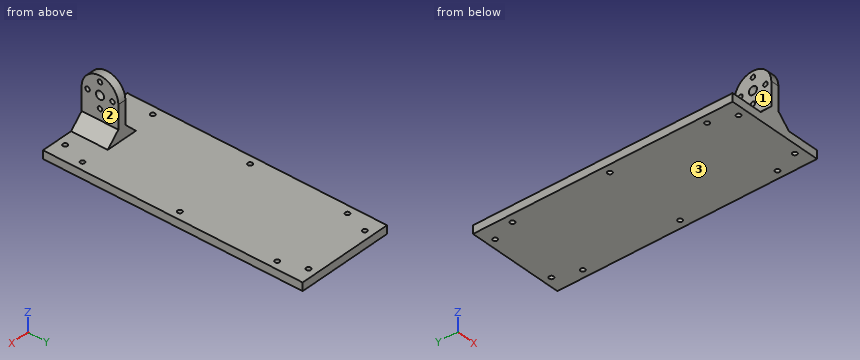
from build123d import *

# Parameters (mm, degrees)
SKETCH1_W           = 76.2
SKETCH1_H           = 203.2
BOSS_EXTRUDE1_DEPTH = 6.35
SKETCH2_W           = 6.35
SKETCH2_H           = 28.702
BOSS_EXTRUDE2_DEPTH = 44.45
SKETCH3_R           = 3.175
CUT_EXTRUDE1_DEPTH  = 6.35
SKETCH4_R           = 1.778
CUT_EXTRUDE2_DEPTH  = 6.35
CIRPATTERN1_COUNT   = 4
CUT_EXTRUDE3_DEPTH  = 6.35
SKETCH6_R           = 1.778
CUT_EXTRUDE4_DEPTH  = 6.35
BOSS_EXTRUDE3_DEPTH = 28.702


with BuildPart() as part:
    # Sketch1 → Boss-Extrude1 (new body)
    with BuildSketch(Plane.XY):
        with Locations((38.1, 101.6)):
            Rectangle(SKETCH1_W, SKETCH1_H)
    extrude(amount=BOSS_EXTRUDE1_DEPTH)

    # Sketch2 → Boss-Extrude2 (add)
    with BuildSketch(Plane.XY.offset(6.35)):
        with Locations((38.1, 14.351)):
            Rectangle(SKETCH2_W, SKETCH2_H)
    extrude(amount=BOSS_EXTRUDE2_DEPTH)

    # Sketch3 → Cut-Extrude1 (cut)
    with BuildSketch(Plane(origin=(41.275, 0, 0), x_dir=(0, 0, -1), z_dir=(1, 0, 0))):
        with Locations((-34.154615714, 14.351)):
            Circle(SKETCH3_R)
    extrude(amount=-CUT_EXTRUDE1_DEPTH, mode=Mode.SUBTRACT)

    # Sketch4 → Cut-Extrude2 (cut)
    with BuildSketch(Plane(origin=(41.275, 0, 0), x_dir=(0, 0, -1), z_dir=(1, 0, 0))):
        with Locations((-43.933615714, 14.351)):
            Circle(SKETCH4_R)
    cut_extrude2 = extrude(amount=-CUT_EXTRUDE2_DEPTH, mode=Mode.SUBTRACT)

    # CirPattern1: Cut-Extrude2 ×4 about axis
    cirpattern1_axis = Axis((0, 14.351, 34.154615714), (1, 0, 0))
    for i in range(1, CIRPATTERN1_COUNT):
        add(cut_extrude2.rotate(cirpattern1_axis, i * 360 / CIRPATTERN1_COUNT), mode=Mode.SUBTRACT)

    # Sketch5 → Cut-Extrude3 (cut)
    with BuildSketch(Plane(origin=(41.275, 0, 0), x_dir=(0, 0, -1), z_dir=(1, 0, 0))):
        with BuildLine():
            ThreePointArc((-34.154615714, 0), (-48.505615714, 14.351), (-34.154615714, 28.702))
            Line((-34.154615714, 28.702), (-50.8, 28.702))
            Line((-50.8, 28.702), (-50.8, 0))
            Line((-50.8, 0), (-34.154615714, 0))
        make_face()
    extrude(amount=-CUT_EXTRUDE3_DEPTH, mode=Mode.SUBTRACT)

    # Sketch6 → Cut-Extrude4 (cut)
    with BuildSketch(Plane(origin=(0, 0, 0), x_dir=(-1, 0, 0), z_dir=(0, 0, -1))):
        with Locations((-63.5, 6.35)):
            Circle(SKETCH6_R)
        with Locations((-12.7, 6.35)):
            Circle(SKETCH6_R)
        with Locations((-6.35, 177.8)):
            Circle(SKETCH6_R)
        with Locations((-6.35, 25.4)):
            Circle(SKETCH6_R)
        with Locations((-69.85, 25.4)):
            Circle(SKETCH6_R)
        with Locations((-69.85, 177.8)):
            Circle(SKETCH6_R)
        with Locations((-63.5, 196.85)):
            Circle(SKETCH6_R)
        with Locations((-12.7, 196.85)):
            Circle(SKETCH6_R)
        with Locations((-6.35, 101.6)):
            Circle(SKETCH6_R)
        with Locations((-69.85, 101.6)):
            Circle(SKETCH6_R)
    extrude(amount=-CUT_EXTRUDE4_DEPTH, mode=Mode.SUBTRACT)

    # Sketch8 → Boss-Extrude3 (add)
    with BuildSketch(Plane.XZ):
        Polygon((41.275, 6.35), (41.275, 15.875), (50.8, 6.35), align=None)
        Polygon((34.925, 6.35), (34.925, 15.875), (25.4, 6.35), align=None)
    extrude(amount=-BOSS_EXTRUDE3_DEPTH)


solid = part.part
Work out the finished part from the listing and answer in its coordinate system (mm). Face numbers are marked on the shaded views. A direction names the side the tool comes from. Coordinates: 2 decimals unless noted, no trailing zeros. Write each loop counter-clockwise with the first axis right and the second up, starting at its lowest first coordinate (ties: lowest second). Pieces come first, ordered by that corner, then holes.
1. Flat-ended cylindrical pins translate along their axes: pin 1 (4.5 mm diameter, centred on y = 24.13, z = 34.15, fed in from -X) (3 decimals); pin 2 (1.5 mm diameter, centred on x = 65, y = 182, fed in from +Z); pin 3 (8.5 mm diameter, centred on y = 13.5, z = 34, fed in from +X) (3 decimals). Find the tip coordinate at first contact, or state that the pin passes through.
Results list:
pin 1: stops at x = 34.925
pin 2: stops at z = 6.35
pin 3: stops at x = 41.275
2. The part is cut by section B-B, the plane x = 21. Write down the section's boundary in (y, z), and give its area (3 significant figures).
Results list:
outline: (0, 0) - (203.2, 0) - (203.2, 6.35) - (0, 6.35) - close
area: 1,290 mm2
3. Consider line 1 along Y through (x, z) = (12.7, 4.75); line 2 along X through (y, z) = (6, 4); line 3 along X through (y, z) = (177.8, 5). Determine where each line is inside the solid, lowest interval first.
Results list:
line 1: y = 0 to 4.57, 8.13 to 195.07, 198.63 to 203.2
line 2: x = 0 to 10.96, 14.44 to 61.76, 65.24 to 76.2
line 3: x = 0 to 4.57, 8.13 to 68.07, 71.63 to 76.2
4. For the marked faces 1, 2 and 3, determine the directions among +Z, -Z, +X, -X, +Y, -Y from which every point of the face is accessible in a straight line to the end or side of a thin tool.
Results list:
face 1: +Z, -X, +Y, -Y
face 2: +Z, +X, +Y, -Y
face 3: -Z, +X, -X, +Y, -Y
5. The part is cut by section A-A, the plane z = 12.5. Write down the section's boundary in (x, y), and give its area (3 significant figures).
Results list:
outline: (31.55, 0) - (44.65, 0) - (44.65, 28.7) - (31.55, 28.7) - close
area: 376 mm2
